Work out the finished part from the listing and answer in its coordinate system (mm). Face numbers are marked on the shaded views. A direction names the side the tool comes from. Round coordinates to 2 decimals unless told otherwise and drop trailing zeros. Write each loop counter-clockwise with the first axis right and the second up, starting at its lowest first coordinate (ties: lowest second). Pieces come first, ordered by that corner, then holes. Notation, with made-up numbers: M 26.5,-24.75 L 79.5,-24.75 A20 cw 79.5,-2.75 Z; hole C 72,9 d5. An arc over 180 degrees is marked long. One line per item, written item: value. Start each with the question number.
Q1. The mould has two halves that part along X. Classify the marked faces 3, 4 and 5: released by +X, released by -X, zero draft, split by the parting line, or undercut.
Q2. A tool of negligible diameter and unlimited length cuts with its end or side. For the marked faces 1 and 2, from which of +Z, -Z, +X, -X, +Y, -Y can it reach the whole face along a straight path? Write none if from no direction.
Q3. Find section A-A (z = 98.5). Write down the section's boundary in (x, y), and give its area (3 significant figures).
Q4. Given pin 1 Ø6 at (x, y) = (106, 107.5) entering from +Z; pin 2 Ø5 at (x, z) = (168.5, 117.5) entering from +Y; pin 3 Ø1 at (y, z) = (33.5, 109.5) entering from -X, each flat-ended and moving along its own axis, determine where each tip first touches the part or whether it passes through.
Q5. Consider probe 1 along X at (y, z) = (119.5, 69.5); probe 2 along X at (y, z) = (33, 118); probe 3 along Z at (x, y) = (110.5, 97). Determine where each line is inside the solid, lowest interval first.
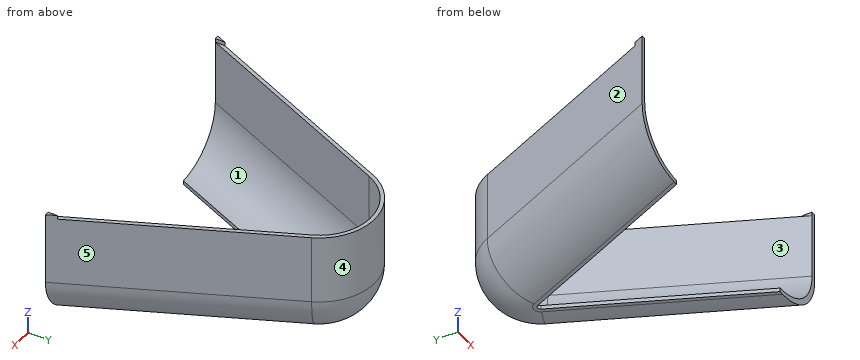
from build123d import *

# Parameters (mm, degrees)
F1_DEPTH = 63.5
F2_T     = -2
F3_R     = 25.4
F4_ANGLE = 180
F5_ANGLE = -48
F6_W     = 145.6223272032
F6_H     = 2
F7_DEPTH = 127
F8_DEPTH = 25.4


# Not quite as in the source:
# - a feature names something its author has since deleted; it is built from what else it names


with BuildPart() as f1:
    # F0 (on Top) → F1 (new body)
    with BuildSketch(Plane.XY):
        with BuildLine():
            Line((-10.2850095064, 143.0450051312), (-58.2692639971, 33.9835022184))
            Line((-58.2692639971, 33.9835022184), (91.7307360029, 34.4206405823))
            Line((91.7307360029, 34.4206405823), (42.7254554371, 143.2713651338))
            ThreePointArc((42.7254554371, 143.2713651338), (44.5808039736, 137.7049772305), (45.2782310553, 131.8791221047))
            Line((45.2782310553, 131.8791221047), (45.4024820726, 131.3612216192))
            Line((45.4024820726, 131.3612216192), (45.2828539684, 131.3612216192))
            ThreePointArc((45.2828539684, 131.3612216192), (16.2705971829, 102.3489648337), (-12.7416596027, 131.3612216192))
            ThreePointArc((-12.7416596027, 131.3612216192), (-12.1208550885, 137.3308515669), (-10.2850095064, 143.0450051312))
        make_face()
        with BuildLine():
            ThreePointArc((42.7254554371, 143.2713651338), (16.1467130657, 160.3732139071), (-10.2850095064, 143.0450051312))
            ThreePointArc((-10.2850095064, 143.0450051312), (-12.1208550885, 137.3308515669), (-12.7416596027, 131.3612216192))
            Line((-12.7416596027, 131.3612216192), (45.2828539684, 131.3612216192))
            ThreePointArc((45.2828539684, 131.3612216192), (45.2816982171, 131.6201821781), (45.2782310553, 131.8791221047))
            ThreePointArc((45.2782310553, 131.8791221047), (44.5808039736, 137.7049772305), (42.7254554371, 143.2713651338))
        make_face()
        with BuildLine():
            Line((45.2828539684, 131.3612216192), (-12.7416596027, 131.3612216192))
            ThreePointArc((-12.7416596027, 131.3612216192), (16.2705971829, 102.3489648337), (45.2828539684, 131.3612216192))
        make_face()
        with BuildLine():
            Line((45.4024820726, 131.3612216192), (45.2782310553, 131.8791221047))
            ThreePointArc((45.2782310553, 131.8791221047), (45.2816982171, 131.6201821781), (45.2828539684, 131.3612216192))
            Line((45.2828539684, 131.3612216192), (45.4024820726, 131.3612216192))
        make_face()
    extrude(amount=F1_DEPTH)

    # F2
    f2_openings = [f1.faces().sort_by_distance(p)[0] for p in [
        (16.730736, 34.202071, 31.75),
    ]]
    offset(amount=F2_T, openings=f2_openings)

    # F3
    f3_edges = [f1.edges().sort_by_distance(p)[0] for p in [
        (16.146713, 160.373214, 63.5),
        (16.155253, 158.373232, 61.5),
    ]]
    fillet(f3_edges, radius=F3_R)


with BuildPart() as f1_1:
    # F4: moved
    add(f1.part.rotate(Axis((41.7381236511, 83.5918491789, 63.5), (-0.4105210981, 0.9118510997, 0)), F4_ANGLE))


with BuildPart() as f1_2:
    # F5: moved
    add(f1_1.part.rotate(Axis((45.4087001389, 13.5661687977, 95.25), (0, 0, 1)), F5_ANGLE))

    # F6 (on face) → F7 (cut)
    with BuildSketch(Plane(origin=(-0.0716524101, 13.3215442397, 0), x_dir=(0.9999855352, 0.0053786087, 0), z_dir=(0.0053786087, -0.9999855352, 0))):
        with Locations((120.4826499572, 126)):
            Rectangle(F6_W, F6_H)
    extrude(amount=-F7_DEPTH, mode=Mode.SUBTRACT)

    # F8 (cut): a face of the model
    f8_faces = [f1_2.faces().sort_by_distance(p)[0] for p in [
        (120.299637411, 47.6367123165, 65.5),
    ]]
    extrude(f8_faces, amount=-F8_DEPTH, mode=Mode.SUBTRACT)


solid = f1_2.part
The answers:
1. face 3: undercut
1. face 4: split by the parting line
1. face 5: released by +X
2. face 1: +Z, -Y
2. face 2: +Z, -Z, -X, +Y
3. outline: M 45.41,13.57 L 47.6,13.58 L 95.34,122.01 A27.01 cw 144.7,122.21 L 193.22,14.36 L 195.41,14.37 L 146.52,123.03 A29.01 ccw 93.51,122.82 Z
3. area: 604 mm2
4. pin 1: z = 68.96
4. pin 2: y = 79.74
4. pin 3: x = 53.96
5. probe 1: 101.89 to 107.26, 132.86 to 138.23
5. probe 2: 53.96 to 56.15, 184.83 to 187.03
5. probe 3: 63.5 to 65.54
